Can you work these out from the model? Positions are in its coordinate system, mm. A direction names the side the tool comes from. Give positions to 0.01 mm unless a question says otherwise; leave off trailing zeros. Order: outer loops, then holes, each group sorted by start corner. A loop starts at its lowest first (then second) coordinate and runs counter-clockwise, first axis right, second up. Notation, with made-up numbers: (-38.75, 57) -> (-26.75, 57) arc R30 ccw to (-26.75, 79) -> close; hole circle Ø3 at (-34.5, -18.5). An arc over 180 degrees is marked (long way). Answer as a JSON object with one key per item and string values.
```python
from build123d import *

# Parameters (mm, degrees)
SKETCH1_W           = 43
SKETCH1_H           = 43
SKETCH1_W_2         = 33
SKETCH1_H_2         = 33
BOSS_EXTRUDE1_DEPTH = 25
SKETCH3_W           = 43
SKETCH3_H           = 43
BOSS_EXTRUDE2_DEPTH = 5
SKETCH4_W           = 20
SKETCH4_H           = 5
BOSS_EXTRUDE3_DEPTH = 30
SKETCH5_R           = 2.25
CUT_EXTRUDE1_DEPTH  = 6
SKETCH_1_W          = 21.5
SKETCH_1_H          = 43
CUT_EXTRUDE_1_DEPTH = 25
SKETCH_3_W          = 25
SKETCH_3_H          = 10
EXTRUDE_1_DEPTH     = 7
FILLET_1_R          = 1
SKETCH_4_R          = 1.6
CUT_EXTRUDE_2_DEPTH = 22.5
CUT_EXTRUDE_3_DEPTH = 3
SKETCH_6_W          = 16.75
SKETCH_6_H          = 33.5
CUT_EXTRUDE_4_DEPTH = 25
FILLET_2_R          = 1
FILLET_3_R          = 1
FILLET_4_R          = 5
FILLET_6_R          = 1
CUT_EXTRUDE_5_DEPTH = 1
SKETCH_9_W          = 5
SKETCH_9_H          = 20
EXTRUDE_2_DEPTH     = 31.5
SKETCH_10_R         = 2.25
CUT_EXTRUDE_6_DEPTH = 6
FILLET_7_R          = 5
FILLET_8_R          = 3
FILLET_9_R          = 1


with BuildPart() as part:
    # Sketch1 → Boss-Extrude1 (new body)
    with BuildSketch(Plane.XY):
        with Locations((16.5, 16.5)):
            Rectangle(SKETCH1_W, SKETCH1_H)
        with Locations((16.5, 16.5)):
            Rectangle(SKETCH1_W_2, SKETCH1_H_2, mode=Mode.SUBTRACT)
    extrude(amount=BOSS_EXTRUDE1_DEPTH)

    # Sketch3 → Boss-Extrude2 (add)
    with BuildSketch(Plane(origin=(0, 0, 0), x_dir=(-1, 0, 0), z_dir=(0, 0, -1))):
        with Locations((-16.5, 16.5)):
            Rectangle(SKETCH3_W, SKETCH3_H)
    extrude(amount=BOSS_EXTRUDE2_DEPTH)

    # Sketch4 → Boss-Extrude3 (add)
    with BuildSketch(Plane(origin=(0, 38, 0), x_dir=(1, 0, 0), z_dir=(0, 1, 0))):
        with Locations((16.5, 2.5)):
            Rectangle(SKETCH4_W, SKETCH4_H)
    boss_extrude3 = extrude(amount=BOSS_EXTRUDE3_DEPTH)

    # Sketch5 → Cut-Extrude1 (cut, through all)
    with BuildSketch(Plane.XY):
        with Locations((16.5, 59.5)):
            Circle(SKETCH5_R)
    cut_extrude1 = extrude(amount=-CUT_EXTRUDE1_DEPTH, mode=Mode.SUBTRACT)

    # Mirror1: Boss-Extrude3, Cut-Extrude1 across plane
    add(boss_extrude3.mirror(Plane(origin=(0, 16.5, 0), x_dir=(0, 0, 1), z_dir=(0, -1, 0))))
    add(cut_extrude1.mirror(Plane(origin=(0, 16.5, 0), x_dir=(0, 0, 1), z_dir=(0, -1, 0))), mode=Mode.SUBTRACT)

    # Эскиз1 → Вырез-Вытянуть1 (cut)
    with BuildSketch(Plane.XY.offset(25)):
        with Locations((5.75, 16.5)):
            Rectangle(SKETCH_1_W, SKETCH_1_H)
    extrude(amount=-CUT_EXTRUDE_1_DEPTH, mode=Mode.SUBTRACT)

    # Эскиз3 → Бобышка-Вытянуть1 (add)
    with BuildSketch(Plane.ZY.offset(-16.5)):
        with Locations((12.5, -10)):
            Rectangle(SKETCH_3_W, SKETCH_3_H)
    extrude_1 = extrude(amount=-EXTRUDE_1_DEPTH)

    # Скругление1
    fillet_1_edges = [part.edges().sort_by_distance(p)[0] for p in [
        (23.5, -5, 12.5),
    ]]
    fillet(fillet_1_edges, radius=FILLET_1_R)

    # Эскиз4 → Вырез-Вытянуть2 (cut, through all)
    with BuildSketch(Plane.ZY.offset(-16.5)):
        with Locations((20, -10)):
            Circle(SKETCH_4_R)
        with Locations((5, -10)):
            Circle(SKETCH_4_R)
    cut_extrude_2 = extrude(amount=-CUT_EXTRUDE_2_DEPTH, mode=Mode.SUBTRACT)

    # Эскиз5 → Вырез-Вытянуть3 (cut)
    with BuildSketch(Plane(origin=(23.5, 0, 0), x_dir=(0, 0, -1), z_dir=(1, 0, 0))):
        Polygon((-18.354551733, -12.85), (-16.709103466, -10), (-18.354551733, -7.15), (-21.645448267, -7.15), (-23.290896534, -10), (-21.645448267, -12.85), align=None)
        Polygon((-6.645448267, -12.85), (-3.354551733, -12.85), (-1.709103466, -10), (-3.354551733, -7.15), (-6.645448267, -7.15), (-8.290896534, -10), align=None)
    cut_extrude_3 = extrude(amount=-CUT_EXTRUDE_3_DEPTH, mode=Mode.SUBTRACT)

    # Зеркальное отражение2: Бобышка-Вытянуть1 across plane
    add(extrude_1.mirror(Plane(origin=(0, 16.5, 0), x_dir=(0, 0, 1), z_dir=(0, -1, 0))))

    # Зеркальное отражение3: Вырез-Вытянуть2 across plane
    add(cut_extrude_2.mirror(Plane(origin=(0, 16.5, 0), x_dir=(0, 0, 1), z_dir=(0, -1, 0))), mode=Mode.SUBTRACT)

    # Зеркальное отражение4: Вырез-Вытянуть3 across plane
    add(cut_extrude_3.mirror(Plane(origin=(0, 16.5, 0), x_dir=(0, 0, 1), z_dir=(0, -1, 0))), mode=Mode.SUBTRACT)

    # Эскиз6 → Вырез-Вытянуть4 (cut)
    with BuildSketch(Plane.XY.offset(25)):
        with Locations((24.875, 16.5)):
            Rectangle(SKETCH_6_W, SKETCH_6_H)
    extrude(amount=-CUT_EXTRUDE_4_DEPTH, mode=Mode.SUBTRACT)

    # Скругление2
    fillet_2_edges = [part.edges().sort_by_distance(p)[0] for p in [
        (23.5, 38, 12.5),
    ]]
    fillet(fillet_2_edges, radius=FILLET_2_R)

    # Скругление3
    fillet_3_edges = [part.edges().sort_by_distance(p)[0] for p in [
        (25.5, -5, 0),
        (23.5, -10.5, 0),
        (23.792893219, -5.292893219, 0),
        (23.5, 43.5, 0),
        (25.5, 38, 0),
        (23.792893219, 38.292893219, 0),
    ]]
    fillet(fillet_3_edges, radius=FILLET_3_R)

    # Скругление4
    fillet_4_edges = [part.edges().sort_by_distance(p)[0] for p in [
        (6.5, -35, -2.5),
        (26.5, -35, -2.5),
        (6.5, 68, -2.5),
        (26.5, 68, -2.5),
    ]]
    fillet(fillet_4_edges, radius=FILLET_4_R)

    # Скругление6
    fillet_6_edges = [part.edges().sort_by_distance(p)[0] for p in [
        (33.25, 33.25, 12.5),
        (33.25, -0.25, 12.5),
        (24.875, 33.25, 0),
        (33.25, 16.5, 0),
        (24.875, -0.25, 0),
    ]]
    fillet(fillet_6_edges, radius=FILLET_6_R)

    # Эскиз7 → Вырез-Вытянуть5 (cut)
    with BuildSketch(Plane.ZY.offset(-16.5)):
        with BuildLine():
            Line((0, 48), (0, 32.25))
            ThreePointArc((0, 32.25), (0.292893219, 32.957106781), (1, 33.25))
            Line((1, 33.25), (25, 33.25))
            Line((25, 33.25), (25, 48))
            Line((25, 48), (0, 48))
        make_face()
        with BuildLine():
            Line((25, -15), (25, -0.25))
            Line((25, -0.25), (1, -0.25))
            ThreePointArc((1, -0.25), (0.292893219, 0.042893219), (0, 0.75))
            Line((0, 0.75), (0, -15))
            Line((0, -15), (25, -15))
        make_face()
    extrude(amount=-CUT_EXTRUDE_5_DEPTH, mode=Mode.SUBTRACT)

    # Эскиз9 → Бобышка-Вытянуть2 (add)
    with BuildSketch(Plane(origin=(38, 0, 0), x_dir=(0, 0, -1), z_dir=(1, 0, 0))):
        with Locations((2.5, 16.5)):
            Rectangle(SKETCH_9_W, SKETCH_9_H)
    extrude(amount=EXTRUDE_2_DEPTH)

    # Эскиз10 → Вырез-Вытянуть6 (cut, through all)
    with BuildSketch(Plane.XY):
        with Locations((59.5, 16.5)):
            Circle(SKETCH_10_R)
    extrude(amount=-CUT_EXTRUDE_6_DEPTH, mode=Mode.SUBTRACT)

    # Скругление7
    fillet_7_edges = [part.edges().sort_by_distance(p)[0] for p in [
        (69.5, 6.5, -2.5),
        (69.5, 26.5, -2.5),
    ]]
    fillet(fillet_7_edges, radius=FILLET_7_R)

    # Скругление8
    fillet_8_edges = [part.edges().sort_by_distance(p)[0] for p in [
        (6.5, -5, -2.5),
        (6.5, 38, -2.5),
        (26.5, 38, -2),
        (26.5, -5, -2),
        (38, 6.5, -2.5),
        (38, 26.5, -2.5),
        (38, 16.5, 0),
    ]]
    fillet(fillet_8_edges, radius=FILLET_8_R)

    # Скругление9
    fillet_9_edges = [part.edges().sort_by_distance(p)[0] for p in [
        (38, -5, 10),
        (38, 38, 10),
    ]]
    fillet(fillet_9_edges, radius=FILLET_9_R)


solid = part.part
```
1. Please list where these lines run through material, in increasing order: L1, parallel to Y at x = 19.45, z = 5; L2, parallel to X at y = -26.5, z = -1.3.
Worked answers:
{"L1": "-15 to -11.6, -8.4 to -0.25, 33.25 to 41.4, 44.6 to 48", "L2": "6.5 to 14.25, 18.75 to 26.5"}
2. Will these pins go through, and if not, where does the flat tip stop? pin 1 Ø0.9 at (x, z) = (21.5, 5) entering from -Y; pin 2 Ø10 at (y, z) = (-10.5, 16) entering from +X; pin 3 Ø7.5 at (x, z) = (22, 10.5) entering from +Y.
Worked answers:
{"pin 1": "y = -15", "pin 2": "x = 23.63", "pin 3": "y = 48"}
3. For faces 1 (the face through (16, -35, -3)), 2 (the face through (25, -0.25, 13)), 3 (the face through (26.5, -19, -2)), 4 (the face through (22.021, 44.405, 7.48)), 5 (the face through (18.98, -11.56, 19.65)), which set-ups out of +Z, -Z, +X, -X, +Y, -Y let a thin tool reach every point of the face, with its end or its side?
Worked answers:
{"face 1": "+Z, -Z, +X, -X, -Y", "face 2": "+Z, -X", "face 3": "+Z, -Z, +X, -Y", "face 4": "+X", "face 5": "+X, -X"}
4. If we mould it in two halves opening along Y, with no side actions, what happens to faces 6 (the face through (22.02, 41.56, 22.46)), 7 (the face through (68, 7.93, -2.54)), 8 (the face through (25, 66.57, -2.54))? For each: +Y half, -Y half, draft (parallel to the pull), parting line (faces both ways), or undercut.
Worked answers:
{"face 6": "undercut", "face 7": "-Y half", "face 8": "+Y half"}
5. If we section it at A-A on x = 59.5: Please give me the cut outline in (y, z).
Worked answers:
{"outline": "(6.5, -5) -> (14.25, -5) -> (14.25, 0) -> (6.5, 0) -> close; (18.75, -5) -> (26.5, -5) -> (26.5, 0) -> (18.75, 0) -> close"}
6. If we section it at B-B on y = 16.5: Please give me the cut outline in (x, z).
Worked answers:
{"outline": "(-5, -5) -> (57.25, -5) -> (57.25, 0) -> (41, 0) arc R3 cw to (38, 3) -> (38, 25) -> (33.25, 25) -> (33.25, 1) arc R1 cw to (32.25, 0) -> (-5, 0) -> close; (61.75, -5) -> (69.5, -5) -> (69.5, 0) -> (61.75, 0) -> close"}
7. If we section it at C-C on z = 4.5: Count the separate pieces of the cut face and the enclosed holes in it, then the cut area to 3 significant figures.
Worked answers:
{"separate pieces": "3", "enclosed holes": "0", "area": "422 mm²"}
8. If we section it at D-D on z = 13.5: Please give me the cut outline in (x, y), then the cut area to 3 significant figures.
Worked answers:
{"outline": "(17.5, -15) -> (23.5, -15) -> (23.5, -6) arc R1 cw to (24.5, -5) -> (37, -5) arc R1 ccw to (38, -4) -> (38, 37) arc R1 ccw to (37, 38) -> (24.5, 38) arc R1 cw to (23.5, 39) -> (23.5, 48) -> (17.5, 48) -> (17.5, 33.25) -> (32.25, 33.25) arc R1 cw to (33.25, 32.25) -> (33.25, 0.75) arc R1 cw to (32.25, -0.25) -> (17.5, -0.25) -> close", "area": "474 mm²"}
